Autodesk Inventor part; units mm, degrees
ref_plane "YZ Plane" through (0, 0, 0) normal (1, 0, 0) x (0, 1, 0)
ref_plane "XZ Plane" through (0, 0, 0) normal (0, 1, 0) x (-1, 0, 0)
ref_plane "XY Plane" through (0, 0, 0) normal (0, 0, 1) x (1, 0, 0)
sketch "스케치1" plane through (0, 0, 0) normal (0, 0, 1) x (1, 0, 0)
  line L0 (0, 17.4) -> (0, -17.4) construction
  line L1 (-20, 17.4) -> (-20, -17.4)
  line L2 (20, -17.4) -> (20, 17.4)
  arc A0 (20, 17.4) -> (-20, 17.4) centre (0, 17.4) ccw
  arc A1 (-20, -17.4) -> (20, -17.4) centre (0, -17.4) ccw
  point P0 (0, 0)
  point P1 (0, 0)
  dimension "d0" = 34.8
  dimension "d1" = 40
extrude "돌출1" add sketch "스케치1" along normal blind 25
sketch "스케치2" plane through (0, 0, 25) normal (0, 0, 1) x (1, 0, 0)
  circle A0 centre (0, 18.7) radius 18.7
  point P0 (0, 0)
  dimension "d4" = 37.4
extrude "돌출2" add sketch "스케치2" along normal blind 145
sketch "스케치3" plane through (0, 18.7, 170) normal (0, 0, 1) x (1, 0, 0)
  circle A0 centre (0, 0) radius 12.5
  point P0 (0, -18.7)
  dimension "d7" = 25
extrude "돌출3" add sketch "스케치3" along normal blind 34
sketch "스케치5" plane through (0, 0, 0) normal (0, 0, -1) x (-1, 0, 0)
  line L0 (-7.5, 8.75) -> (7.5, 8.75)
  line L1 (7.5, 8.75) -> (7.5, 26.05)
  line L2 (7.5, 26.05) -> (-7.5, 26.05)
  line L3 (-7.5, 26.05) -> (-7.5, 8.75)
  arc A0 (20, 17.4) -> (-20, 17.4) centre (0, 17.4) ccw
  point P0 (0, 0)
  dimension "d10" = 15
  dimension "d11" = 17.3
  dimension "d12" = 8.65
  dimension "d13" = 7.5
extrude "돌출4" add sketch "스케치5" along normal blind 19
sketch "스케치6" plane through (-20, -17.4, 0) normal (-1, 0, 0) x (0, 0, 1)
  circle A0 centre (-10, 34.8) radius 3
  line L0 (-19, 26.15) -> (-19, 43.45)
  line L1 (0, 43.45) -> (-19, 43.45)
  circle A1 centre (195, 34.8) radius 3
  line L2 (0, 0) -> (25, 0)
  point P0 (0, 17.4)
  dimension "d16" = 6
  dimension "d17" = 9
  dimension "d18" = 8.65
  dimension "d19" = 205
  dimension "d20" = 34.8
  dimension "d21" = 6
extrude "돌출5" cut sketch "스케치6" against normal through all
sketch "스케치7" plane through (0, 0, 25) normal (0, 0, 1) x (1, 0, 0)
  circle A0 centre (0, -17.8723) radius 19
  circle A1 centre (0, 18.7) radius 18.7
  point P0 (0, 0)
  point P1 (-37.4551, 11.4874)
  point P2 (4.5758, 0.5685)
  point P3 (-4.5758, 0.5685)
  dimension "d25" = 38
  dimension "d26" = 0
extrude "돌출6" add sketch "스케치7" along normal blind 80 contours A0 A1 picked at (-1.0542, -24.4512)
properties part number "높이조절 액추에이터_최소" material "알루미늄 6061"
The model under review builds one solid part; all positions refer to its coordinate system, in mm. A direction names the side the tool comes from. Round coordinates to 2 decimals unless told otherwise and drop trailing zeros. Loops run counter-clockwise (first coordinate to the right, second up) from the corner with the lowest first, then second, coordinate; pieces in that order, holes last. Notation, with made-up numbers: (-36, -37.5) -> (4, -37.5) arc R21 ccw to (4, -27.5) -> close; hole circle Ø1 at (24, -39.5). An arc over 180 degrees is marked (long way). Write item = value, one per line. Start each with the question number.
Item 1: Insertion check: pin 1 (3 mm diameter, centred on x = -4, z = 64, fed in from +Y); pin 2 (12 mm diameter, centred on x = -2, z = -8.5, fed in from +Y); pin 3 (2 mm diameter, centred on x = 2, y = -6, fed in from -Z); pin 4 (5 mm diameter, centred on y = 17.4, z = 195, fed in from +X). Each pin has a flat end and moves straight along its axis. Give the tip position at first contact, or say it passes through.
Item 2: Take a section at C-C on z = 18.5. Give the boundary of the cut face in (x, y).
Item 3: For faces 5 (the flat face through (7.5, 16, -7)), 6 (the flat face through (12.2, 14.8, 170)), 7 (the cylindrical face through (0.44, -37.395, 12.325)), 8 (the flat face through (-7.5, 19, -7)), list the 3-axis set-ups (+Z, -Z, +X, -X, +Y, -Y) from which the entire face can be reached by the end or side of a thin tool; tool diameter is ignored.
Item 4: To check wall thickness, follow L1, parallel to Z at x = 3, y = 17; L2, parallel to Z at x = -10.5, y = 17; L3, parallel to Y at x = 3, z = -10. State the ranges of each line that lie inside material, in increasing order.
Item 5: Mouldability with a two-part tool opening along Y and no side actions: class faces 1 (the cylindrical face through (-4.054, 36.955, 96.485)), 2 (the cylindrical face through (0.771, -36.857, 64.44)), 3 (the cylindrical face through (-2.71, 30.903, 186.762)), 4 (the flat face through (0, 26.05, -9)) as released by +Y, released by -Y, zero draft, split by the parting line, or undercut.
Item 6: Take a section at A-A on z = -10. Give the boundary of the cut face in (x, y).
Item 7: Take a section at B-B on y = -5. Give the boundary of the cut face in (x, z).
Item 8: Take a section at D-D on y = 11. Give the boundary of the cut face in (x, z), plus the area to 3 significant figures.
Result:
q1.pin_1 = 37.23
q1.pin_2 = 26.05
q1.pin_3 = 0
q1.pin_4 = through
q2.outline = (-20, -17.4) arc R20 ccw to (20, -17.4) -> (20, 17.4) arc R20 ccw to (-20, 17.4) -> close
q3.face_5 = -Z, +X, +Y, -Y
q3.face_6 = +Z
q3.face_7 = +Z, -Z, -Y
q3.face_8 = -Z, -X, +Y, -Y
q4.L1 = -19 to -12.97, -7.03 to 192.03, 197.97 to 204
q4.L2 = 0 to 192.03, 197.97 to 204
q4.L3 = 8.75 to 14.4, 20.4 to 26.05
q5.face_1 = undercut
q5.face_2 = undercut
q5.face_3 = split by the parting line
q5.face_4 = released by +Y
q6.outline = (-7.5, 8.75) -> (7.5, 8.75) -> (7.5, 14.4) -> (-7.5, 14.4) -> close; (-7.5, 20.4) -> (7.5, 20.4) -> (7.5, 26.05) -> (-7.5, 26.05) -> close
q7.outline = (-20, 0) -> (20, 0) -> (20, 25) -> (13.98, 25) -> (13.98, 105) -> (-13.98, 105) -> (-13.98, 25) -> (-20, 25) -> close
q8.outline = (-20, 0) -> (-7.5, 0) -> (-7.5, -19) -> (7.5, -19) -> (7.5, 0) -> (20, 0) -> (20, 25) -> (17.04, 25) -> (17.04, 170) -> (9.85, 170) -> (9.85, 204) -> (-9.85, 204) -> (-9.85, 170) -> (-17.04, 170) -> (-17.04, 25) -> (-20, 25) -> close
q8.area = 6,900 mm²
